```python
from build123d import *

# Parameters (mm, degrees)
SKETCH_2_W          = 20
SKETCH_2_H          = 11
EXTRUDE_1_DEPTH     = 14
SKETCH_4_R          = 1.6
CUT_EXTRUDE_1_DEPTH = 21
SKETCH_5_R          = 1.5
CUT_EXTRUDE_2_DEPTH = 2.9


with BuildPart() as part:
    # 草图2 → 凸台-拉伸1 (new body)
    with BuildSketch(Plane.XY):
        Rectangle(SKETCH_2_W, SKETCH_2_H)
    extrude(amount=-EXTRUDE_1_DEPTH)

    # 草图4 → 切除-拉伸1 (cut, through all)
    with BuildSketch(Plane(origin=(10, 0, 0), x_dir=(0, 0, -1), z_dir=(1, 0, 0))):
        with BuildLine():
            ThreePointArc((6.1, -2.5), (4.5, -0.9), (2.9, -2.5))
            Line((2.9, -2.5), (2.9, -5.5))
            Line((2.9, -5.5), (6.1, -5.5))
            Line((6.1, -5.5), (6.1, -2.5))
        make_face()
        with BuildLine():
            Line((2.9, 5.5), (2.9, 2.5))
            ThreePointArc((2.9, 2.5), (4.5, 0.9), (6.1, 2.5))
            Line((6.1, 2.5), (6.1, 5.5))
            Line((6.1, 5.5), (2.9, 5.5))
        make_face()
        with Locations((11, 0)):
            Circle(SKETCH_4_R)
    extrude(amount=-CUT_EXTRUDE_1_DEPTH, mode=Mode.SUBTRACT)

    # 草图5 → 切除-拉伸2 (cut)
    with BuildSketch(Plane.XY):
        with Locations((-5, 0)):
            Circle(SKETCH_5_R)
        with Locations((5, 0)):
            Circle(SKETCH_5_R)
    extrude(amount=-CUT_EXTRUDE_2_DEPTH, mode=Mode.SUBTRACT)


solid = part.part
```
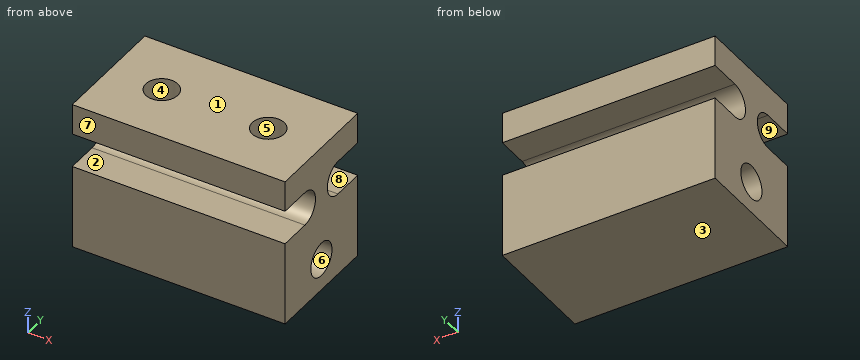
Can you work these out from the model? Positions are in its coordinate system, mm. Face numbers are marked on the shaded views. A direction names the side the tool comes from. Give positions to 0.01 mm unless a question says otherwise; leave off trailing zeros. Order: outer loops, then holes, each group sorted by start corner. A loop starts at its lowest first (then second) coordinate and runs counter-clockwise, first axis right, second up. Notation, with made-up numbers: M 53,89.5 L 86,89.5 A13 cw 86,93.5 Z; hole C 56,-39 d11. An arc over 180 degrees is marked long. One line per item, written item: value.
1) I want a section at A-A, the plane x = -1. List the corners of the cut face in (y, z) for me.
Answer sheet:
outline: M -5.5,-14 L 5.5,-14 L 5.5,-6.1 L 2.5,-6.1 A1.6 cw 2.5,-2.9 L 5.5,-2.9 L 5.5,0 L -5.5,0 L -5.5,-2.9 L -2.5,-2.9 A1.6 cw -2.5,-6.1 L -5.5,-6.1 Z; hole C 0,-11 d3.2
2) Please list where these lines run through material, in increasing order: line 1 along Z through (x, y) = (0, 4.25); line 2 along Y through (x, z) = (4.25, -11); line 3 along Z through (x, y) = (5, -1.25).
Answer sheet:
line 1: z = -14 to -6.1, -2.9 to 0
line 2: y = -5.5 to -1.6, 1.6 to 5.5
line 3: z = -14 to -12, -10 to -5.5, -3.5 to -2.9
3) On a 3-axis mill with a long thin cutter (end or side, diameter ignored), from which of +Z, -Z, +X, -X, +Y, -Y can I reach the whole of each face in a straight line? I mean the marked faces 5, 6, 7, 8 and 9. Say none if no direction works.
Answer sheet:
face 5: +Z
face 6: +X, -X
face 7: +Z, -Z, +X, -X, -Y
face 8: +X, -X, +Y
face 9: +X, -X, -Y
4) I want a section at B-B, the plane y = 3.25. List the corners of the cut face in (x, z) for me.
Answer sheet:
outline: M -10,-14 L 10,-14 L 10,-6.1 L -10,-6.1 Z; M -10,-2.9 L 10,-2.9 L 10,0 L -10,0 Z
5) For P1, Ø2.5, axis at x = 5, y = 0, coming from the +Z side, with a flat end and sliding along its axis, tell me the tip position at first contact or that it passes through.
Answer sheet:
P1: stops at z = -2.9
6) I want a section at D-D, the plane y = 0. List the corners of the cut face in (x, z) for me, plus the area to 3 significant figures.
Answer sheet:
outline: M -10,-14 L 10,-14 L 10,-12.6 L -10,-12.6 Z; M -10,-9.4 L 10,-9.4 L 10,0 L 6.5,0 L 6.5,-2.9 L 3.5,-2.9 L 3.5,0 L -3.5,0 L -3.5,-2.9 L -6.5,-2.9 L -6.5,0 L -10,0 Z
area: 199 mm^2
7) We'd pull the mould along Z, two halves only. Please class the marked faces 1, 2, 3 and 4: released by +Z, released by -Z, zero draft, split by the parting line, or undercut.
Answer sheet:
face 1: released by +Z
face 2: undercut
face 3: released by -Z
face 4: zero draft
8) I want a section at C-C, the plane z = -11. List the corners of the cut face in (x, y) for me.
Answer sheet:
outline: M -10,-5.5 L 10,-5.5 L 10,-1.6 L -10,-1.6 Z; M -10,1.6 L 10,1.6 L 10,5.5 L -10,5.5 Z
